Geometry: final body of the model. Coordinates: model frame, mm. A direction names the side the tool comes from. Round coordinates to 2 decimals unless told otherwise and drop trailing zeros. Loops run counter-clockwise (first coordinate to the right, second up) from the corner with the lowest first, then second, coordinate; pieces in that order, holes last. Notation, with made-up numbers: M -18,59.25 L 25,59.25 A23 cw 25,93.25 Z; hole C 87.5,25 d11. An arc over 180 degrees is marked long. Return JSON: item names as keys, results as strings.
Autodesk Inventor part; units mm, degrees
ref_plane "YZ Plane" through (0, 0, 0) normal (1, 0, 0) x (0, 1, 0)
ref_plane "XZ Plane" through (0, 0, 0) normal (0, 1, 0) x (-1, 0, 0)
ref_plane "XY Plane" through (0, 0, 0) normal (0, 0, 1) x (1, 0, 0)
sketch "Эскиз1" plane through (0, 0, 0) normal (0, 1, 0) x (-1, 0, 0)
  line L0 (0, 9.5) -> (0, 14.5)
  line L1 (0, 14.5) -> (-2, 14.5)
  line L2 (-2, 14.5) -> (-2, 28)
  line L3 (-55, 4) -> (-55, 8)
  line L4 (-55, 8) -> (-52, 8)
  line L5 (-10, 28) -> (-10, 13)
  line L6 (-10, 13) -> (-47, 13)
  line L7 (-2, 14.5) -> (-2, 28)
  line L8 (-2, 28) -> (-10, 28)
  line L9 (-52, 8) -> (-47.3096, 12.6904)
  line L10 (-47.3096, 12.6904) -> (-47, 13)
  line L11 (0, 0) -> (0, 9.5)
  line L12 (0, 9.5) -> (-2, 9.5)
  line L13 (-2, 7.5) -> (-2, 9.5)
  line L14 (-2, 7.5) -> (-5.5, 7.5)
  line L15 (-5.5, 7.5) -> (-5.5, 9)
  line L16 (-5.5, 9) -> (-8, 9)
  line L17 (0, 0) -> (0, 7)
  line L18 (-8, 9) -> (-8, 0)
  line L19 (-30, 0) -> (-30, 8)
  line L20 (-30, 8) -> (-42, 8)
  line L21 (-42, 8) -> (-42, 6)
  line L22 (-55, 4) -> (-44, 4)
  line L23 (-42, 6) -> (-44, 4)
  line L24 (0, 0) -> (-55, 0)
  line L25 (-8, 0) -> (-30, 0)
  point P0 (-42, 4)
  dimension "d26" = 30
  dimension "d27" = 12
  dimension "d28" = 2
  dimension "d29" = 2
  dimension "d30" = 55
  dimension "d31" = 8
  dimension "d32" = 16
  dimension "d33" = 26
  dimension "d34" = 16
  dimension "d35" = 12
  dimension "d36" = 42
  dimension "d37" = 18
  dimension "d38" = 8
  dimension "d39" = 2.5
  dimension "d40" = 29
  dimension "d41" = 19
  dimension "d42" = 15
  dimension "d43" = 2
  dimension "d44" = 55
  dimension "d45" = 3
  dimension "d46" = 135
  dimension "d47" = 45
  dimension "d48" = 56
  dimension "d49" = 2
revolve "Вращение1" add sketch "Эскиз1" angle 360 about axis through (0, 0, 0) along (1, 0, 0) contours L12 L13 L14 L15 L16 L18 L24 L19 L20 L21 L23 L22 L3 L4 L9 L10 L6 L5 L8 L2 L1 L0
sketch "Эскиз3" plane through (8, 0, 0) normal (-1, 0, 0) x (0, 0, 1)
  point P0 (0, 0)
  point P1 (0, 0)
hole "Отверстие2" at (8, 0, 0) direction (1, 0, 0) diameter 12.376 depth 30
sketch "Эскиз4" plane through (2, 0, 0) normal (-1, 0, 0) x (0, 0, 1)
  circle A0 centre (0, 0) radius 21
  point P0 (0, 21)
  dimension "d65" = 42
chamfer "Фаска1" distance 2 angle 45 1 edges at (8, 0, -6.188)
sketch "Эскиз5" plane through (2, 0, 0) normal (-1, 0, 0) x (0, 0, 1)
  point P0 (0, 0)
hole "Отверстие4" at (2, 21, 0) direction (1, 0, 0) diameter 9 depth 30
pattern_circular "Круговой массив2" count 3 over 360 about axis through (1, 0, 0) along (-1, 0, 0) of "Отверстие4"
sketch "Эскиз6" plane through (2, 0, 0) normal (-1, 0, 0) x (0, 0, 1)
  circle A0 centre (0, 0) radius 28
  line L0 (55.1219, -20) -> (-57.0995, -20)
  line L1 (55.1219, -20) -> (-57.0995, -20)
  line L2 (-57.0995, -20) -> (-57.0995, -35.8887)
  line L3 (-57.0995, -35.8887) -> (55.1219, -35.8887)
  line L4 (55.1219, -35.8887) -> (55.1219, -20)
  point P0 (0, 28)
  point P1 (19.5959, -20)
  point P2 (-19.5959, -20)
  dimension "d91" = 48
extrude "Выдавливание1" cut sketch "Эскиз6" against normal blind 10 contours L0 A0 picked at (4.9079, -21.2721)
Q1. Section query B-B (z = 0). State how many separate pieces and enclosed holes the cut face has, plus the area to 3 significant figures.
Determined:
{"separate pieces": "3", "enclosed holes": "0", "area": "773 mm^2"}
Q2. Section query A-A (y = 21). Output: boundary loops of the cut face in (x, z).
Determined:
{"outline": "M 2,-18.52 L 10,-18.52 L 10,-4.5 L 2,-4.5 Z; M 2,4.5 L 10,4.5 L 10,18.52 L 2,18.52 Z"}
Q3. Pull-direction query (Z, two-part tool) for faces 1 (the flat face through (55, 2, -4)), 2 (the flat face through (8, 8, 3)), 3 (the cylindrical face through (53.48, -7.81, -1.73)); classes: pulls with the +Z half, pulls with the -Z half, needs draft (parallel to the pull), parting line crosses it, or undercut.
Determined:
{"face 1": "needs draft", "face 2": "undercut", "face 3": "parting line crosses it"}
Q4. Reachability of faces 4 (the cylindrical face through (6.06, -14.96, -18.77)), 5 (the conical face through (9.875, -6.163, -1.369)), 6 (the flat face through (10, 14, 0)), 7 (the cylindrical face through (1.014, 12.864, 6.691)) from +Z, -Z, +X, -X, +Y, -Y: full face, straight path, thin tool, end or side. Return the list, or none.
Determined:
{"face 4": "+X, -X", "face 5": "none", "face 6": "+X", "face 7": "-X"}
Q5. Material intervals for L1, parallel to Z at x = 7, y = 0; L2, parallel to X at y = -1, z = 18; L3, parallel to X at y = 13.5, z = 4.5, sorted ascending.
Determined:
{"L1": "z = -28 to -9, 9 to 28", "L2": "x = 2 to 10", "L3": "x = 0 to 10"}
Q6. Section query C-C (x = 40). Output: boundary loops of the cut face in (y, z).
Determined:
{"outline": "C 0,0 d26; hole C 0,0 d16"}
Q7. Pin query (flat end, axial travel): pin 1 (2 mm diameter, centred on x = 16, y = -14.5, fed in from -Z); pin 2 (1.5 mm diameter, centred on y = 4, z = -7, fed in from -X); pin 3 (8 mm diameter, centred on x = 24.5, y = 13.5, fed in from -Z); pin 4 (14.5 mm diameter, centred on y = 0, z = 0, fed in from -X). Return the tip coordinate at first contact, or that it passes through.
Determined:
{"pin 1": "passes through", "pin 2": "stops at x = 2", "pin 3": "stops at z = -8.87", "pin 4": "stops at x = 8.94"}
